Solid Edge part; units mm, degrees
sketch "Sketch1" plane through (0, 0, 0) normal (0, -1, 0) x (1, 0, 0)
  line L0 (-15, -24) -> (15, -24)
  line L1 (15, -24) -> (15, 24)
  line L2 (15, 24) -> (-15, 24)
  line L3 (-15, 24) -> (-15, -24)
  dimension "D1" = 15
  dimension "D2" = 15
extrude "Protrusion1" add sketch "Sketch1" along normal mid plane 5
sketch "Sketch2" plane through (0, -2.5, 0) normal (0, -1, 0) x (1, 0, 0)
  circle A0 centre (0, 0) radius 12
extrude "Extrusionsausschnitt_1" cut sketch "Sketch2" against normal blind 310
hole "Bohrung_1" at (-10, 0, 24) direction (0, 0, -1) diameter 3.5 depth 8
hole "Hole1" at (10, 0, 24) direction (0, 0, -1) diameter 3.5 depth 8
mirror "Mirror1" about plane through (0, 0, 0) normal (0, 0, 1) of "Bohrung_1", "Hole1"
properties material "Aluminiumlegierung:3.0205, Al 99.0, EN-AW 1200"
Build history of the part. All positions in model axes, mm. A direction names the side the tool comes from. Coordinates: 2 decimals unless noted, no trailing zeros. Order: outer loops, then holes, each group sorted by start corner. A loop starts at its lowest first (then second) coordinate and runs counter-clockwise, first axis right, second up. Notation, with made-up numbers: M -11.75,7 L 42.25,7 A19 cw 42.25,31 Z; hole C -29.75,36.25 d2. An arc over 180 degrees is marked long. One line per question, with ' | ' between items. Start each with the question number.
1. Wall check: line 1 along X through (y, z) = (0, -18.25); line 2 along Y through (x, z) = (-10, 19.75); line 3 along Z through (x, y) = (0, 0). Give the ranges that are in metal, low to high. Write a range as [from, to].
2. Tool access for faces 1 (the face through (10, 0, -16)), 2 (the face through (-11.735, 0.228, 19.944)), 3 (the face through (-11.99, -0.04, 0.53)): list every direction of +Z, -Z, +X, -X, +Y, -Y with a clear straight run to the whole face (end or side of a thin tool).
3. Mould opens along Y. For faces 4 (the face through (0, 0, -24)), 5 (the face through (7, 2.5, 11)), 6 (the face through (8.265, 0.228, 19.944)) say: +Y half, -Y half, draft (parallel to the pull), parting line (faces both ways), or undercut.
4. Cut at C-C (x = 10). Write the cut outline in (y, z).
5. Cut at B-B (z = 0). Write the cut outline in (x, y), plus the area to 3 significant figures.
6. Cut at D-D (z = 18). Write the cut outline in (x, y), plus the area to 3 significant figures.
7. Flat gauge pins, fed straight in: P1, Ø3, axis at x = -10, y = 0, coming from the -Z side; P2, Ø1.8, axis at x = -10.5, y = 0.5, coming from the +Z side. Where does each tip first touch, or does it go through?
8. Cut at A-A (y = 0). Write the cut outline in (x, z).
The answers:
1) line 1: x = [-15, -11.75], [-8.25, 8.25], [11.75, 15] | line 2: y = [-2.5, -1.75], [1.75, 2.5] | line 3: z = [-24, -12], [12, 24]
2) face 1: -Z | face 2: +Z | face 3: +Y, -Y
3) face 4: draft | face 5: +Y half | face 6: undercut
4) outline: M -2.5,-24 L -1.75,-24 L -1.75,-16 L 1.75,-16 L 1.75,-24 L 2.5,-24 L 2.5,-6.63 L -2.5,-6.63 Z; M -2.5,6.63 L 2.5,6.63 L 2.5,24 L 1.75,24 L 1.75,16 L -1.75,16 L -1.75,24 L -2.5,24 Z
5) outline: M -15,-2.5 L -12,-2.5 L -12,2.5 L -15,2.5 Z; M 12,-2.5 L 15,-2.5 L 15,2.5 L 12,2.5 Z | area: 30.0 mm2
6) outline: M -15,-2.5 L 15,-2.5 L 15,2.5 L -15,2.5 Z; hole C -10,0 d3.5; hole C 10,0 d3.5 | area: 131 mm2
7) P1: stops at z = -16 | P2: stops at z = 16
8) outline: M -15,-24 L -11.75,-24 L -11.75,-16 L -8.25,-16 L -8.25,-24 L 8.25,-24 L 8.25,-16 L 11.75,-16 L 11.75,-24 L 15,-24 L 15,24 L 11.75,24 L 11.75,16 L 8.25,16 L 8.25,24 L -8.25,24 L -8.25,16 L -11.75,16 L -11.75,24 L -15,24 Z; hole C 0,0 d24
